```python
from build123d import *

# Parameters (mm, degrees)
F0_W      = 25
F0_H      = 5
F0_W_2    = 6.9
F0_H_2    = 2
F1_DEPTH  = 40
F2_W      = 25
F2_H      = 5
F3_DEPTH  = 1
F4_W      = 25
F4_H      = 5
F5_DEPTH  = 10.25
F6_W      = 25
F6_H      = 5
F7_DEPTH  = 36
F8_W      = 25
F8_H      = 2
F9_DEPTH  = 26
F10_W     = 25
F10_H     = 2
F11_DEPTH = 24


with BuildPart() as f1:
    # F0 (on Front) → F1 (new body)
    with BuildSketch(Plane.XZ):
        with Locations((0.35389, 1)):
            Rectangle(F0_W, F0_H)
        with Locations((-6.44611, 1)):
            Rectangle(F0_W_2, F0_H_2, mode=Mode.SUBTRACT)
        with Locations((6.95389, 1)):
            Rectangle(F0_W_2, F0_H_2, mode=Mode.SUBTRACT)
    extrude(amount=F1_DEPTH)

    # F2 (on face) → F3 (join)
    with BuildSketch(Plane.XZ.offset(40)):
        with Locations((0.35389, 1)):
            Rectangle(F2_W, F2_H)
    extrude(amount=F3_DEPTH)

    # F4 (on face) → F5 (join)
    with BuildSketch(Plane(origin=(0, 0, -1.5), x_dir=(1, 0, 0), z_dir=(0, 0, -1))):
        with Locations((0.35389, 2.5)):
            Rectangle(F4_W, F4_H)
    extrude(amount=F5_DEPTH)

    # F6 (on face) → F7 (join)
    with BuildSketch(Plane.XZ.offset(5)):
        with Locations((0.35389, -9.25)):
            Rectangle(F6_W, F6_H)
    extrude(amount=F7_DEPTH)

    # F8 (on face) → F9 (join)
    with BuildSketch(Plane.XY.offset(3.5)):
        with Locations((0.35389, -25)):
            Rectangle(F8_W, F8_H)
    extrude(amount=F9_DEPTH)

    # F10 (on face) → F11 (join)
    with BuildSketch(Plane(origin=(0, -24, 0), x_dir=(-1, 0, 0), z_dir=(0, 1, 0))):
        with Locations((-0.35389, 28.5)):
            Rectangle(F10_W, F10_H)
    extrude(amount=F11_DEPTH)


solid = f1.part
```
The model under review builds one solid part; all positions refer to its coordinate system, in mm. A direction names the side the tool comes from. Round coordinates to 2 decimals unless told otherwise and drop trailing zeros. Loops run counter-clockwise (first coordinate to the right, second up) from the corner with the lowest first, then second, coordinate; pieces in that order, holes last.
Item 1: Take a section at D-D (y = -3.5). Write out the cut boundary in (x, z), then the cut area to 3 significant figures.
Determined:
outline: (-12.15, -11.75) - (12.85, -11.75) - (12.85, 3.5) - (-12.15, 3.5) - close; (-12.15, 27.5) - (12.85, 27.5) - (12.85, 29.5) - (-12.15, 29.5) - close; hole (-9.9, 0) - (-3, 0) - (-3, 2) - (-9.9, 2) - close; hole (3.5, 0) - (10.4, 0) - (10.4, 2) - (3.5, 2) - close
area: 404 mm2
Item 2: Mouldability with a two-part tool opening along X and no side actions: class faces 1 (the face through (0, -41, -9)), 2 (the face through (7, -20, 0)), 3 (the face through (12.854, -18, 0)) as released by +X, released by -X, zero draft, split by the parting line, or undercut.
Determined:
face 1: zero draft
face 2: undercut
face 3: released by +X
Item 3: Take a section at C-C (x = -2). Write out the cut boundary in (y, z).
Determined:
outline: (-41, -11.75) - (0, -11.75) - (0, 3.5) - (-24, 3.5) - (-24, 27.5) - (0, 27.5) - (0, 29.5) - (-26, 29.5) - (-26, 3.5) - (-41, 3.5) - (-41, -1.5) - (-5, -1.5) - (-5, -6.75) - (-41, -6.75) - close
Item 4: Take a section at B-B (y = -14). Write out the cut boundary in (x, z), then the cut area to 3 significant figures.
Determined:
outline: (-12.15, -11.75) - (12.85, -11.75) - (12.85, -6.75) - (-12.15, -6.75) - close; (-12.15, -1.5) - (12.85, -1.5) - (12.85, 3.5) - (-12.15, 3.5) - close; (-12.15, 27.5) - (12.85, 27.5) - (12.85, 29.5) - (-12.15, 29.5) - close; hole (-9.9, 0) - (-3, 0) - (-3, 2) - (-9.9, 2) - close; hole (3.5, 0) - (10.4, 0) - (10.4, 2) - (3.5, 2) - close
area: 272 mm2
Item 5: Take a section at A-A (y = -36). Write out the cut boundary in (x, z), then the cut area to 3 significant figures.
Determined:
outline: (-12.15, -11.75) - (12.85, -11.75) - (12.85, -6.75) - (-12.15, -6.75) - close; (-12.15, -1.5) - (12.85, -1.5) - (12.85, 3.5) - (-12.15, 3.5) - close; hole (-9.9, 0) - (-3, 0) - (-3, 2) - (-9.9, 2) - close; hole (3.5, 0) - (10.4, 0) - (10.4, 2) - (3.5, 2) - close
area: 222 mm2
Item 6: For line 1 (Z direction, x = 0.5, y = -23); line 2 (Z direction, x = -7.25, y = -8); line 3 (Z direction, x = 8, y = -3), list the stretches that pass through material, from the lowest coordinate up.
Determined:
line 1: z = -11.75 to -6.75, -1.5 to 3.5, 27.5 to 29.5
line 2: z = -11.75 to -6.75, -1.5 to 0, 2 to 3.5, 27.5 to 29.5
line 3: z = -11.75 to 0, 2 to 3.5, 27.5 to 29.5
Item 7: Clearance check with flat-ended pins moving along their axes: pin 1 Ø5 at (y, z) = (-12.5, 23.5) entering from +X; pin 2 Ø12 at (x, z) = (-5, 11) entering from +Y; pin 3 Ø1.6 at (x, z) = (7, 1) entering from +Y; pin 4 Ø12 at (x, y) = (0, -34) entering from +Z. State where each tip first meets the part, or that it passes through.
Determined:
pin 1: passes through
pin 2: stops at y = -24
pin 3: stops at y = -40
pin 4: stops at z = 3.5
Item 8: For faces 4 (the face through (0, -23, -6.75)), 5 (the face through (0, -33, 3.5)), 6 (the face through (-9.896, -20, 1)), 7 (the face through (0, -12, 3.5)), list the 3-axis set-ups (+Z, -Z, +X, -X, +Y, -Y) from which the entire face can be reached by the end or side of a thin tool; tool diameter is ignored.
Determined:
face 4: +X, -X, -Y
face 5: +Z, +X, -X, -Y
face 6: +Y
face 7: +X, -X, +Y
